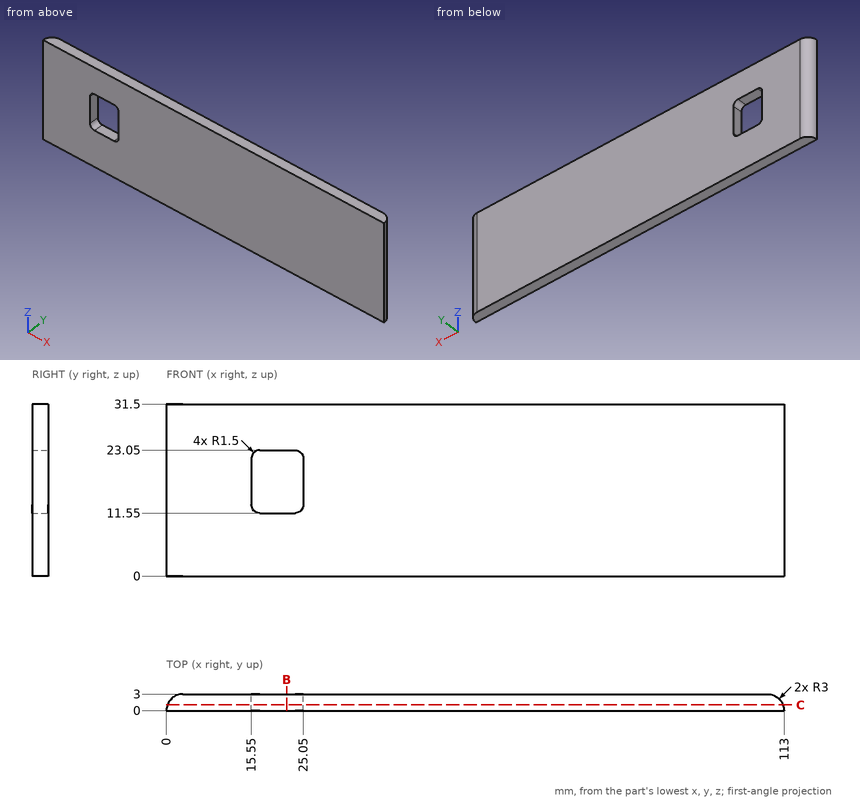
Study the drawing (mm; zero at the part's minimum x, y, z) and answer. Coordinates: 2 decimals unless noted, no trailing zeros. Write each loop counter-clockwise with the first axis right and the second up, starting at its lowest first coordinate (ties: lowest second). Pieces come first, ordered by that corner, then holes. Notation, with made-up numbers: (62.5, -15.75) - (114.5, -15.75) arc R32 ccw to (114.5, 15.25) - close; hole circle Ø11 at (-38, 22.25). An arc over 180 degrees is marked (long way). Answer as a JSON object with one key per item and string values. Group by question number.
1. A cutting plane is placed at C-C (y = 1.05). Determine the outline of the cut face in (x, z), plus the area to 3 significant figures.
2. A cutting plane is placed at B-B (x = 22). Determine the outline of the cut face in (y, z).
3. Consider L1, parallel to Z at x = 19, y = 1.2; L2, parallel to X at y = 0.2, z = 9; L3, parallel to X at y = 2.15, z = 16.5. Determine where each line is inside the solid, lowest interval first. Write a range as [from, to].
4. Each of these flat-tipped pins is pushed along its axis until it touches: P1, Ø1.5, axis at y = 2, z = 18.5, coming from the +X side; P2, Ø1.5, axis at y = 2.5, z = 13.5, coming from the +X side. Where does it stop, or does it pass through?
Worked out:
{
 "1": {"outline": "(0.19, 0) - (112.81, 0) - (112.81, 31.5) - (0.19, 31.5) - close; hole (15.55, 13.05) arc R1.5 ccw to (17.05, 11.55) - (23.55, 11.55) arc R1.5 ccw to (25.05, 13.05) - (25.05, 21.55) arc R1.5 ccw to (23.55, 23.05) - (17.05, 23.05) arc R1.5 ccw to (15.55, 21.55) - close", "area": "3,440 mm²"},
 "2": {"outline": "(0, 0) - (3, 0) - (3, 11.55) - (0, 11.55) - close; (0, 23.05) - (3, 23.05) - (3, 31.5) - (0, 31.5) - close"},
 "3": {"L1": "z = [0, 11.55], [23.05, 31.5]", "L2": "x = [0.01, 112.99]", "L3": "x = [0.91, 15.55], [25.05, 112.09]"},
 "4": {"P1": "stops at x = 112.73", "P2": "stops at x = 112.44"}
}
